from build123d import *

# Parameters (mm, degrees)
F0_R     = 28.575532
F1_DEPTH = 40.2336
F2_DEPTH = 40.2336
F3_R     = 3.302
F4_R     = 10.162681
F5_DEPTH = 15.7734


with BuildPart() as f1:
    # F0 (on Top) → F1 (new body)
    with BuildSketch(Plane.XY):
        with Locations((-45.395139, 0)):
            Circle(F0_R)
        with BuildLine():
            Line((-26.875399, 4.833719), (-26.875399, 0))
            Line((-26.875399, 0), (-26.875399, -4.835614))
            Line((-26.875399, -4.835614), (-31.951214, -4.835614))
            ThreePointArc((-31.951214, -4.835614), (-59.682276, 0.001007), (-31.950532, 4.833719))
            Line((-31.950532, 4.833719), (-26.875399, 4.833719))
        make_face(mode=Mode.SUBTRACT)
        with BuildLine():
            Line((-39.865061, 4.833719), (-31.950532, 4.833719))
            ThreePointArc((-31.950532, 4.833719), (-59.682276, 0.001007), (-31.951214, -4.835614))
            Line((-31.951214, -4.835614), (-39.865061, -4.835614))
            Line((-39.865061, -4.835614), (-39.865061, 0))
            Line((-39.865061, 0), (-39.865061, 4.833719))
        make_face()
    extrude(amount=F1_DEPTH)

    # F0 (on Top) → F2 (cut)
    with BuildSketch(Plane.XY):
        with BuildLine():
            Line((-31.108002, 0), (-26.875399, 0))
            Line((-26.875399, 0), (-26.875399, 4.833719))
            Line((-26.875399, 4.833719), (-31.950532, 4.833719))
            ThreePointArc((-31.950532, 4.833719), (-31.320211, 2.453298), (-31.108002, 0))
        make_face()
        with BuildLine():
            Line((-39.865061, 4.833719), (-31.950532, 4.833719))
            ThreePointArc((-31.950532, 4.833719), (-59.682276, 0.001007), (-31.951214, -4.835614))
            Line((-31.951214, -4.835614), (-39.865061, -4.835614))
            Line((-39.865061, -4.835614), (-39.865061, 0))
            Line((-39.865061, 0), (-39.865061, 4.833719))
        make_face()
    extrude(amount=F2_DEPTH, mode=Mode.SUBTRACT)

    # F3
    f3_edges = [f1.edges().sort_by_distance(p)[0] for p in [
        (-73.970671, 0, 40.2336),
    ]]
    fillet(f3_edges, radius=F3_R)

    # F4 (on Top) → F5 (join)
    with BuildSketch(Plane.XY):
        with BuildLine():
            Line((8.595701, 19.046027), (-26.525037, 22.033167))
            Line((-26.525037, 22.033167), (-26.240665, -21.475879))
            Line((-26.240665, -21.475879), (8.595701, -19.046027))
            ThreePointArc((8.595701, -19.046027), (27.641729, 0), (8.595701, 19.046027))
        make_face()
        with Locations((8.595701, 0)):
            Circle(F4_R, mode=Mode.SUBTRACT)
    extrude(amount=F5_DEPTH)


solid = f1.part
Model file for the job. Use its own axes, mm. A direction names the side the tool comes from. Give positions to 0.01 mm unless a question says otherwise; leave off trailing zeros. Order: outer loops, then holes, each group sorted by start corner. A loop starts at its lowest first (then second) coordinate and runs counter-clockwise, first axis right, second up. Notation, with made-up numbers: (-2.5, -17.75) - (17.5, -17.75) arc R33 cw to (17.5, 10.25) - close; hole circle Ø5 at (83, -10). An arc over 180 degrees is marked (long way). One line per item, written item: value.
Item 1: Pin check, flat tips, straight feed: pin 1 Ø1.5 at (x, z) = (-60.5, 5) entering from +Y; pin 2 Ø8 at (y, z) = (-9.5, 23.5) entering from +X; pin 3 Ø3 at (x, y) = (-50.5, 11.5) entering from +Z; pin 4 Ø7.5 at (y, z) = (1, 10.5) entering from -X. Stop position of each tip, or through.
Response values:
pin 1: y = 24.71
pin 2: x = -17.35
pin 3: through
pin 4: x = -73.97
Item 2: Slice it at A-A (z = 5). List the corners of the cut face in (x, y).
Response values:
outline: (-26.53, 22.03) - (-26.52, 21.46) arc R28.58 ccw (long way) to (-26.24, -21.21) - (-26.24, -21.48) - (8.6, -19.05) arc R19.05 ccw to (8.6, 19.05) - close; hole (-31.95, -4.84) - (-26.88, -4.84) - (-26.88, 4.83) - (-31.95, 4.83) arc R14.29 ccw (long way) to start; hole circle Ø20.33 at (8.6, 0)
Item 3: Slice it at C-C (z = 27). List the corners of the cut face in (x, y).
Response values:
outline: circle Ø57.15 at (-45.4, 0); hole (-31.95, -4.84) - (-26.88, -4.84) - (-26.88, 4.83) - (-31.95, 4.83) arc R14.29 ccw (long way) to start
Item 4: Wall check: line 1 (X direction, y = 6, z = 10); line 2 (X direction, y = 6.5, z = 4); line 3 (X direction, y = 0, z = 27). Give the ranges that are in metal, low to high.
Response values:
line 1: -73.33 to -58.36, -32.43 to 0.39, 16.8 to 26.67
line 2: -73.22 to -58.12, -32.67 to 0.78, 16.41 to 26.5
line 3: -73.97 to -59.68, -26.88 to -16.82
Item 5: Tool access for faces 4 (the cylindrical face through (27.637, -0.419, 7.776)), 5 (the flat face through (-29, -4.836, 20)), 6 (the cylindrical face through (-73.943, 1.256, 18.207)): list every direction of +Z, -Z, +X, -X, +Y, -Y with a clear straight run to the whole face (end or side of a thin tool).
Response values:
face 4: +Z, -Z, +X
face 5: +Z, -Z
face 6: +Z
Item 6: Slice it at D-D (y = 7). Give the number of separate pieces and of enclosed holes in the cut face, then the cut area to 3 significant figures.
Response values:
separate pieces: 3
enclosed holes: 0
area: 1,680 mm2
Item 7: Two-plate mould, pull along Y, no slides. Class faces 1 (the flat face through (-9.07, -20.28, 7.78)), 2 (the flat face through (-26.875, 0, 20)), 3 (the flat face through (-6, 1, 15.773)): released by +Y, released by -Y, zero draft, split by the parting line, or undercut.
Response values:
face 1: released by -Y
face 2: undercut
face 3: zero draft
Item 8: Slice it at B-B (y = 0). List the corners of the cut face in (x, z).
Response values:
outline: (-73.97, 0) - (-59.68, 0) - (-59.68, 40.23) - (-70.67, 40.23) arc R3.3 ccw to (-73.97, 36.93) - close; (-26.88, 0) - (-1.57, 0) - (-1.57, 15.77) - (-16.82, 15.77) - (-16.82, 36.93) arc R3.3 ccw to (-20.12, 40.23) - (-26.88, 40.23) - close; (18.76, 0) - (27.64, 0) - (27.64, 15.77) - (18.76, 15.77) - close
